The model under review builds one solid part; all positions refer to its coordinate system, in mm. Round coordinates to 2 decimals unless told otherwise and drop trailing zeros. Write each loop counter-clockwise with the first axis right and the second up, starting at its lowest first coordinate (ties: lowest second). Pieces come first, ordered by that corner, then holes. Notation, with made-up numbers: M 87.5,89 L 95.5,89 A28 cw 95.5,118 Z; hole C 50,-5.5 d8. An arc over 180 degrees is marked long. Write item = value, one per line. Start each with the question number.
Item 1: Take a section at B-B, the plane z = 6.75. Give the boundary of the cut face in (x, y).
Item 2: For pin 1 Ø2 at (y, z) = (-9.5, 6) entering from +X; pin 2 Ø1 at (y, z) = (-1.5, 6.5) entering from -X; pin 3 Ø1 at (y, z) = (-5, 6) entering from +X; pin 4 Ø0.6 at (x, y) = (0.5, -8) entering from +Z, all flat-tipped, find the tip position at first contact; note any pin that passes through.
Item 3: To check wall thickness, follow line 1 along X through (y, z) = (-6.37, 0.75); line 2 along Y through (x, z) = (0, -5.5); line 3 along Z through (x, y) = (15, -8.25). State the ranges of each line that lie inside material, in increasing order.
Item 4: Take a section at C-C, the plane y = -9.5. Give the boundary of the cut face in (x, z), plus the area to 3 significant figures.
Item 5: Take a section at A-A, the plane x = -15. Give the boundary of the cut face in (y, z).
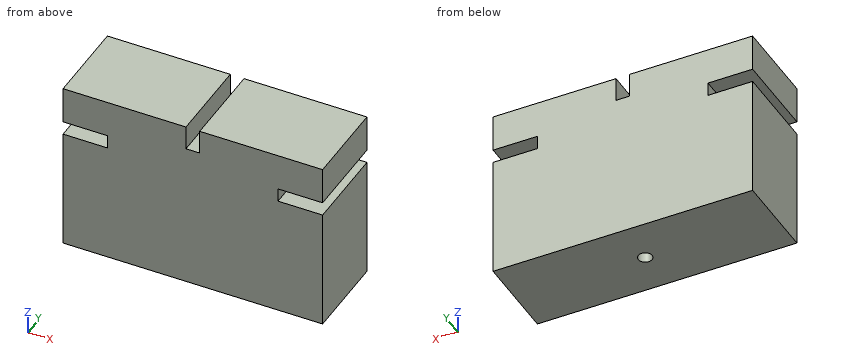
from build123d import *

# Parameters (mm, degrees)
F1_DEPTH = 12.6
F2_R     = 1
F3_DEPTH = 22
F5_DEPTH = 31.301


# Not quite as in the source:
# - a feature names something its author has since deleted; it is built from what else it names


with BuildPart() as f1:
    # F0 (on Front) → F1 (new body)
    with BuildSketch(Plane.XZ):
        Polygon((-1, 12.61), (-18.9, 12.61), (-18.9, 7.19), (-12.4, 7.19), (-12.4, 5.19), (-18.9, 5.19), (-18.9, -12.61), (18.9, -12.61), (18.9, 5.19), (12.4, 5.19), (12.4, 7.19), (18.9, 7.19), (18.9, 12.61), (1, 12.61), (1, 9.06), (0, 9.06), (-1, 9.06), align=None)
    extrude(amount=F1_DEPTH)

    # F2 (on face) → F3 (cut)
    with BuildSketch(Plane(origin=(0, 0, -12.61), x_dir=(1, 0, 0), z_dir=(0, 0, -1))):
        with Locations((0, 6.37)):
            Circle(F2_R)
    extrude(amount=-F3_DEPTH, mode=Mode.SUBTRACT)

    # F4 (on face) → F5 (cut, through all)
    with BuildSketch(Plane(origin=(-12.4, 0, 0), x_dir=(0, -1, 0), z_dir=(-1, 0, 0))):
        with BuildLine():
            ThreePointArc((6.3, 5.19), (7.0071067812, 5.4828932188), (7.3, 6.19))
            ThreePointArc((7.3, 6.19), (7.0071067812, 6.8971067812), (6.3, 7.19))
            ThreePointArc((6.3, 7.19), (5.3, 6.19), (6.3, 5.19))
        make_face()
    extrude(amount=-F5_DEPTH, mode=Mode.SUBTRACT)


solid = f1.part
Response values:
q1.outline = M -12.4,-12.6 L 12.4,-12.6 L 12.4,-7.13 L 0.65,-7.13 A1 cw -0.65,-7.13 L -12.4,-7.13 Z; M -12.4,-5.47 L -0.44,-5.47 A1 cw 0.44,-5.47 L 12.4,-5.47 L 12.4,0 L -12.4,0 Z
q2.pin_1 = 18.9
q2.pin_2 = -12.4
q2.pin_3 = 12.4
q2.pin_4 = 9.06
q3.line_1 = -18.9 to -1, 1 to 18.9
q3.line_2 = -12.6 to -7.37, -5.37 to 0
q3.line_3 = -12.61 to 5.19, 7.19 to 12.61
q4.outline = M -18.9,-12.61 L 18.9,-12.61 L 18.9,5.19 L 12.4,5.19 L 12.4,7.19 L 18.9,7.19 L 18.9,12.61 L 1,12.61 L 1,9.06 L -1,9.06 L -1,12.61 L -18.9,12.61 L -18.9,7.19 L -12.4,7.19 L -12.4,5.19 L -18.9,5.19 Z
q4.area = 920 mm2
q5.outline = M -12.6,-12.61 L 0,-12.61 L 0,5.19 L -12.6,5.19 Z; M -12.6,7.19 L 0,7.19 L 0,12.61 L -12.6,12.61 Z
